Source: CAD feature listing. Evaluate the final solid. Frame: model axes, mm. Face numbers are marked on the shaded views. A direction names the side the tool comes from. Coordinates: 2 decimals unless noted, no trailing zeros. Write each loop counter-clockwise with the first axis right and the second up, starting at its lowest first coordinate (ties: lowest second). Pieces come first, ordered by that corner, then holes. Notation, with made-up numbers: (75.25, -27) - (115.25, -27) arc R29 cw to (115.25, -1) - close; hole circle Ø5 at (49, 60.5). An arc over 180 degrees is marked (long way). One line per question, with ' | ' between items. Start each with the question number.
Q1. Contact query for flat-ended pins moving along their axis: P1, Ø5, axis at y = -1.5, z = 5, coming from the +X side; P2, Ø2, axis at x = 4.37, z = 0, coming from the -Y side. Output: stop coordinate, or through.
Q2. Cut plane A-A, the plane z = 0. Return loops of the section in (x, y) (3 decimals), plus the area to 3 significant figures.
Q3. Draft query along Z for the marked faces 1, 2 and 3. Return one class per face: +Z half, -Z half, draft (parallel to the pull), parting line (faces both ways), or undercut.
Q4. Line query: line 1 (X direction, y = -5, z = 0); line 2 (Z direction, x = 5.25, y = 1.5) (1 decimal); line 3 (Z direction, x = 3, y = -0.75). Output: solid intervals per line, ascending.
Q5. Cut plane C-C, the plane x = 1. Give the number of separate pieces and of enclosed holes in the cut face, plus the area to 3 significant figures.
Q6. Cut plane D-D, the plane y = -6.5. Return loops of the section in (x, z), plus the area to 3 significant figures.
Q7. Cut plane B-B, the plane y = 3. Return loops of the section in (x, z).
Q8. Access query for the marked faces 4, 5 and 6. Directions: +Z, -Z, +X, -X, +Y, -Y. A direction counts if a zero-diameter tool reaches every point of the face in a straight line with its end or side. Return the directions, or none.
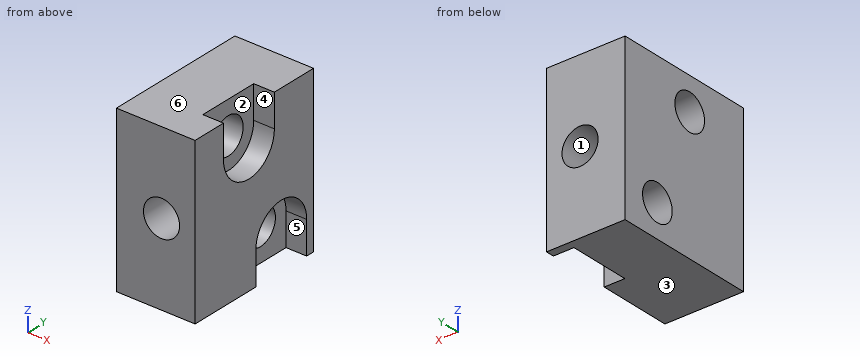
```python
from build123d import *

# Parameters (mm, degrees)
SKETCH1_W           = 11.43
SKETCH1_H           = 15.875
BOSS_EXTRUDE1_DEPTH = 7.62
SKETCH3_R           = 1.75
CUT_EXTRUDE1_DEPTH  = 22.2885
SKETCH4_R           = 1.75
CUT_EXTRUDE2_DEPTH  = 22.2885
SKETCH5_R           = 3
SKETCH5_R_2         = 1.75
CUT_EXTRUDE3_DEPTH  = 2
SKETCH6_W           = 2.54
SKETCH6_H           = 15.875
BOSS_EXTRUDE2_DEPTH = 7.62
CUT_EXTRUDE4_START  = -18.796
SKETCH8_R           = 1.75
CUT_EXTRUDE4_DEPTH  = 18.796


with BuildPart() as part:
    # Sketch1 → Boss-Extrude1 (new body)
    with BuildSketch(Plane.YZ):
        Rectangle(SKETCH1_W, SKETCH1_H)
    extrude(amount=BOSS_EXTRUDE1_DEPTH)

    # Sketch3 → Cut-Extrude1 (cut)
    with BuildSketch(Plane.XZ.offset(5.715)):
        with Locations(Location((4.36625, 0, 0), (0, 0, 270))):
            Circle(SKETCH3_R)
    extrude(amount=-CUT_EXTRUDE1_DEPTH, mode=Mode.SUBTRACT)

    # Sketch4 → Cut-Extrude2 (cut)
    with BuildSketch(Plane.YZ.offset(7.62)):
        with Locations(Location((-1.905, 4.7625, 0), (0, 0, 270))):
            Circle(SKETCH4_R)
        with Locations(Location((1.905, -4.7625, 0), (0, 0, 270))):
            Circle(SKETCH4_R)
    extrude(amount=-CUT_EXTRUDE2_DEPTH, mode=Mode.SUBTRACT)

    # Sketch5 → Cut-Extrude3 (cut)
    # profile 1 of 4: a face of its own
    with BuildSketch(Plane.YZ.offset(7.62)):
        with Locations((-1.905, 4.7625)):
            Circle(SKETCH5_R)
        with Locations(Location((-1.905, 4.7625, 0), (0, 0, 270))):
            Circle(SKETCH5_R_2, mode=Mode.SUBTRACT)
    # profile 2 of 4: a face of its own
    with BuildSketch(Plane.YZ.offset(7.62)):
        with BuildLine():
            Line((-4.905, 7.9375), (-4.905, 4.7625))
            ThreePointArc((-4.905, 4.7625), (-1.905, 7.7625), (1.095, 4.7625))
            Line((1.095, 4.7625), (1.095, 7.9375))
            Line((1.095, 7.9375), (-4.905, 7.9375))
        make_face()
    # profile 3 of 4: a face of its own
    with BuildSketch(Plane.YZ.offset(7.62)):
        with Locations((1.905, -4.7625)):
            Circle(SKETCH5_R)
        with Locations(Location((1.905, -4.7625, 0), (0, 0, 270))):
            Circle(SKETCH5_R_2, mode=Mode.SUBTRACT)
    # profile 4 of 4: a face of its own
    with BuildSketch(Plane.YZ.offset(7.62)):
        with BuildLine():
            Line((4.905, -7.9375), (4.905, -4.7625))
            ThreePointArc((4.905, -4.7625), (1.905, -7.7625), (-1.095, -4.7625))
            Line((-1.095, -4.7625), (-1.095, -7.9375))
            Line((-1.095, -7.9375), (4.905, -7.9375))
        make_face()
    extrude(amount=-CUT_EXTRUDE3_DEPTH, mode=Mode.SUBTRACT)

    # Sketch6 → Boss-Extrude2 (add)
    with BuildSketch(Plane.YZ.offset(7.62)):
        with Locations((-6.985, 0)):
            Rectangle(SKETCH6_W, SKETCH6_H)
    extrude(amount=-BOSS_EXTRUDE2_DEPTH)

    # Sketch8 → Cut-Extrude4 (cut)
    with BuildSketch(Plane(origin=(0, 5.715, 0), x_dir=(-1, 0, 0), z_dir=(0, 1, 0)).offset(CUT_EXTRUDE4_START)):
        with Locations(Location((-4.36625, 0, 0), (0, 0, 270))):
            Circle(SKETCH8_R)
    extrude(amount=CUT_EXTRUDE4_DEPTH, mode=Mode.SUBTRACT)


solid = part.part
```
Reply:
1) P1: stops at x = 5.62 | P2: passes through
2) outline: (0, -8.255) - (2.616, -8.255) - (2.616, 5.715) - (0, 5.715) - close; (6.116, -8.255) - (7.62, -8.255) - (7.62, 5.715) - (6.116, 5.715) - close | area: 57.6 mm^2
3) face 1: undercut | face 2: draft | face 3: -Z half
4) line 1: x = 0 to 2.62, 6.12 to 7.62 | line 2: z = -7.9 to -6.5, -3.1 to -1.5, 1.5 to 7.9 | line 3: z = -7.94 to -1.09, 1.09 to 3.45, 6.08 to 7.94
5) separate pieces: 1 | enclosed holes: 2 | area: 203 mm^2
6) outline: (0, -7.94) - (7.62, -7.94) - (7.62, 7.94) - (0, 7.94) - close; hole circle Ø3.5 at (4.37, 0) | area: 111 mm^2
7) outline: (0, -7.94) - (5.62, -7.94) - (5.62, -6.13) - (0, -6.13) - close; (0, -3.4) - (5.62, -3.4) - (5.62, -1.97) - (7.62, -1.97) - (7.62, 7.94) - (0, 7.94) - close; hole circle Ø3.5 at (4.37, 0)
8) face 4: +Z, +X | face 5: -Z, +X | face 6: +Z, +X, -X, +Y, -Y
